from build123d import *

# Parameters (mm, degrees)
ESQUISSE1_W                  = 12
ESQUISSE1_H                  = 12
BOSS_EXTRU_1_DEPTH           = 15
ENL_V_START                  = -3
ESQUISSE2_R                  = 2.6
ENL_V_MAT_EXTRU_1_DEPTH      = 51.706317156
ENL_V_MAT_EXTRU_1_TAPER      = 2
ESQUISSE3_W                  = 8
ESQUISSE3_H                  = 8
ENL_V_MAT_EXTRU_2_DEPTH      = 13
CHANFREIN1_SIZE              = 1
ESQUISSE4_W                  = 15
ESQUISSE4_H                  = 3
BOSS_EXTRU_2_DEPTH           = 8
ESQUISSE5_R                  = 1.6
ENL_V_MAT_EXTRU_3_DEPTH      = 46.588944696
CHANFREIN2_SIZE              = 0.5
CHANFREIN2_OF_SYM_TRIE1_SIZE = 0.5


with BuildPart() as part:
    # Esquisse1 → Boss.-Extru.1 (new body)
    with BuildSketch(Plane.XY):
        with Locations((-28.630410255, 23.182655502)):
            Rectangle(ESQUISSE1_W, ESQUISSE1_H)
    extrude(amount=BOSS_EXTRU_1_DEPTH)

    # Esquisse2 → Enlèv. mat.-Extru.1 (cut, through all)
    with BuildSketch(Plane.XY.offset(15).offset(ENL_V_START)):
        with Locations((-28.630410255, 23.182655502)):
            Circle(ESQUISSE2_R)
    extrude(amount=ENL_V_MAT_EXTRU_1_DEPTH, taper=ENL_V_MAT_EXTRU_1_TAPER, mode=Mode.SUBTRACT)

    # Esquisse3 → Enlèv. mat.-Extru.2 (cut)
    with BuildSketch(Plane(origin=(0, 0, 0), x_dir=(-1, 0, 0), z_dir=(0, 0, -1))):
        with Locations((28.630410255, 23.182655502)):
            Rectangle(ESQUISSE3_W, ESQUISSE3_H)
    extrude(amount=-ENL_V_MAT_EXTRU_2_DEPTH, mode=Mode.SUBTRACT)

    # Chanfrein1
    chanfrein1_edges = [part.edges().sort_by_distance(p)[0] for p in [
        (-34.630410255, 29.182655502, 7.5),
        (-22.630410255, 29.182655502, 7.5),
        (-22.630410255, 17.182655502, 7.5),
        (-34.630410255, 17.182655502, 7.5),
    ]]
    chamfer(chanfrein1_edges, length=CHANFREIN1_SIZE)

    # Esquisse4 → Boss.-Extru.2 (add)
    with BuildSketch(Plane.ZY.offset(34.630410255)):
        with Locations((7.5, 24.682655502)):
            Rectangle(ESQUISSE4_W, ESQUISSE4_H)
    boss_extru_2 = extrude(amount=BOSS_EXTRU_2_DEPTH)

    # Esquisse5 → Enlèv. mat.-Extru.3 (cut, through all)
    with BuildSketch(Plane.XZ.offset(-23.182655502)):
        with Locations((-38.880410255, 7.5)):
            Circle(ESQUISSE5_R)
    enl_v_mat_extru_3 = extrude(amount=-ENL_V_MAT_EXTRU_3_DEPTH, mode=Mode.SUBTRACT)

    # Chanfrein2
    chanfrein2_edges = [part.edges().sort_by_distance(p)[0] for p in [
        (-42.630410255, 24.682655502, 15),
        (-42.630410255, 24.682655502, 0),
    ]]
    chamfer(chanfrein2_edges, length=CHANFREIN2_SIZE)

    # Symétrie1: Boss.-Extru.2, Enlèv. mat.-Extru.3 across plane
    add(boss_extru_2.mirror(Plane.ZY.offset(28.630410255)))
    add(enl_v_mat_extru_3.mirror(Plane.ZY.offset(28.630410255)), mode=Mode.SUBTRACT)

    # Chanfrein2 of Symétrie1
    chanfrein2_of_sym_trie1_edges = [part.edges().sort_by_distance(p)[0] for p in [
        (-14.630410255, 24.682655502, 15),
        (-14.630410255, 24.682655502, 0),
    ]]
    chamfer(chanfrein2_of_sym_trie1_edges, length=CHANFREIN2_OF_SYM_TRIE1_SIZE)


solid = part.part
Source: CAD feature listing. Evaluate the final solid. Frame: model axes, mm. A direction names the side the tool comes from. Coordinates: 2 decimals unless noted, no trailing zeros. Order: outer loops, then holes, each group sorted by start corner. A loop starts at its lowest first (then second) coordinate and runs counter-clockwise, first axis right, second up.
Item 1: Pull-direction query (Z, two-part tool) for faces 1 (the face through (-37.4, 24.66, 6.89)), 2 (the face through (-29, 29.183, 7)), 3 (the face through (-30.495, 24.892, 14.014)); classes: pulls with the +Z half, pulls with the -Z half, needs draft (parallel to the pull), parting line crosses it, or undercut.
Output values:
face 1: undercut
face 2: needs draft
face 3: pulls with the -Z half
Item 2: Cut plane D-D (z = 5.25). Return loops of the section in (x, y).
Output values:
outline: (-42.63, 23.18) - (-34.63, 23.18) - (-34.63, 18.18) - (-33.63, 17.18) - (-23.63, 17.18) - (-22.63, 18.18) - (-22.63, 23.18) - (-14.63, 23.18) - (-14.63, 26.18) - (-22.63, 26.18) - (-22.63, 28.18) - (-23.63, 29.18) - (-33.63, 29.18) - (-34.63, 28.18) - (-34.63, 26.18) - (-42.63, 26.18) - close; hole (-32.63, 19.18) - (-24.63, 19.18) - (-24.63, 27.18) - (-32.63, 27.18) - close
Item 3: Set-up query: faces 4 (the face through (-34.63, 21, 7)), 5 (the face through (-22.63, 21, 7)), 6 (the face through (-29, 27.183, 6)). Return all of +Z, -Z, +X, -X, +Y, -Y with unobstructed straight access to the full face (end or side cutting, diameter ignored); none if empty.
Output values:
face 4: +Z, -Z, -X, -Y
face 5: +Z, -Z, +X, -Y
face 6: -Z
Item 4: Cut plane B-B (x = -18.25). Return loops of the section in (y, z), plus the area to 3 significant figures.
Output values:
outline: (23.18, 0) - (26.18, 0) - (26.18, 5.91) - (23.18, 5.91) - close; (23.18, 9.09) - (26.18, 9.09) - (26.18, 15) - (23.18, 15) - close
area: 35.4 mm2
Item 5: Material intervals for line 1 (X direction, y = 26, z = 2.5); line 2 (Y direction, x = -28, z = 8.75); line 3 (Z direction, x = -25.5, y = 20.25), sorted ascending.
Output values:
line 1: x = -42.63 to -32.63, -24.63 to -14.63
line 2: y = 17.18 to 19.18, 27.18 to 29.18
line 3: z = 13 to 15
Item 6: Cut plane A-A (z = 7.5). Return loops of the section in (x, y), plus the area to 3 significant figures.
Output values:
outline: (-42.63, 23.18) - (-40.48, 23.18) - (-40.48, 26.18) - (-42.63, 26.18) - close; (-37.28, 23.18) - (-34.63, 23.18) - (-34.63, 18.18) - (-33.63, 17.18) - (-23.63, 17.18) - (-22.63, 18.18) - (-22.63, 23.18) - (-19.98, 23.18) - (-19.98, 26.18) - (-22.63, 26.18) - (-22.63, 28.18) - (-23.63, 29.18) - (-33.63, 29.18) - (-34.63, 28.18) - (-34.63, 26.18) - (-37.28, 26.18) - close; (-16.78, 23.18) - (-14.63, 23.18) - (-14.63, 26.18) - (-16.78, 26.18) - close; hole (-32.63, 19.18) - (-24.63, 19.18) - (-24.63, 27.18) - (-32.63, 27.18) - close
area: 107 mm2
Item 7: Cut plane C-C (y = 26.75). Return loops of the section in (x, z), plus the area to 3 significant figures.
Output values:
outline: (-34.63, 0) - (-32.63, 0) - (-32.63, 13) - (-24.63, 13) - (-24.63, 0) - (-22.63, 0) - (-22.63, 15) - (-34.63, 15) - close
area: 76.0 mm2
Item 8: First-contact query: P1, Ø9, axis at x = -40, z = 7, coming from the +Y side; P2, Ø2.5, axis at x = -20.5, z = 9, coming from the -Y side; P3, Ø2.5, axis at x = -27.5, y = 24, coming from the -Z side. Flat tips, straight axial feed; report the tip coordinate or a pass-through.
Output values:
P1: stops at y = 26.18
P2: stops at y = 23.18
P3: stops at z = 13
